The listing builds one solid part. Answer for the finished solid, in the listing's coordinates (mm). Give positions to 0.01 mm unless a question says otherwise; leave off trailing zeros. Loops run counter-clockwise (first coordinate to the right, second up) from the corner with the lowest first, then second, coordinate; pieces in that order, holes last.
Item 1: Consider line 1 along Z through (x, y) = (24.5, 1.4); line 2 along X through (y, z) = (2.2, 25); line 3 along Z through (x, y) = (26.5, 2). Determine where each line is inside the solid, lowest interval first.
Item 2: Section A-A, the plane z = -22 is taken. Give the vertices of the cut face in (x, y), and give its area (3 significant figures).
Item 3: Each of these flat-tipped pins is pushed along its axis until it touches: pin 1 Ø1 at (y, z) = (2.5, -5) entering from -X; pin 2 Ø2 at (y, z) = (2.5, 9.5) entering from +X; pin 3 Ø3 at (y, z) = (4, 6) entering from +X. Where does it stop, or does it pass through?
Item 4: Section C-C, the plane y = 3 is taken. Give the number of separate pieces and of enclosed holes in the cut face, and give its area (3 significant figures).
Item 5: The mould has two halves that part along Z. Classify faces 1 (the face through (-12.87, 2.58, -33.15)), 2 (the face through (-9, 5.08, -1)), 3 (the face through (-0.768, 2.576, -7.313)), 4 (the face through (29.18, 2.5, -31.83)): pulls with the +Z half, pulls with the -Z half, needs draft (parallel to the pull), parting line crosses it, or undercut.
Item 6: Section B-B, the plane x = 13 is taken. Give the vertices of the cut face in (y, z).
from build123d import *

# Parameters (mm, degrees)
SKETCH2_R           = 43.18
BOSS_EXTRUDE1_DEPTH = 5.08
CUT_EXTRUDE1_DEPTH  = 62.276677456
CUT_EXTRUDE2_DEPTH  = 62.276677456
SKETCH6_R           = 1.016
CUT_EXTRUDE3_DEPTH  = 62.276677456


with BuildPart() as part:
    # Sketch2 → Boss-Extrude1 (new body)
    with BuildSketch(Plane(origin=(0, 0, 0), x_dir=(1, 0, 0), z_dir=(0, 1, 0))):
        with Locations(Location((0, 0, 0), (0, 0, 270))):
            Circle(SKETCH2_R)
    extrude(amount=BOSS_EXTRUDE1_DEPTH)

    # Sketch3 → Cut-Extrude1 (cut, through all)
    with BuildSketch(Plane(origin=(0, 5.08, 0), x_dir=(1, 0, 0), z_dir=(0, 1, 0))):
        with BuildLine():
            Line((1.626393556, 2.3495), (-1.626393556, 2.3495))
            ThreePointArc((-1.626393556, 2.3495), (-1.326251609, -2.531079398), (2.8575, 0))
            ThreePointArc((2.8575, 0), (2.531079398, 1.326251609), (1.626393556, 2.3495))
        make_face()
    extrude(amount=-CUT_EXTRUDE1_DEPTH, mode=Mode.SUBTRACT)

    # Sketch5 → Cut-Extrude2 (cut, through all)
    with BuildSketch(Plane(origin=(0, 5.08, 0), x_dir=(1, 0, 0), z_dir=(0, 1, 0))):
        with BuildLine():
            Line((-9.058813318, 2.943386871), (-33.819569719, 10.98864432))
            ThreePointArc((-33.819569719, 10.98864432), (-35.492818655, -2.184816682), (-32.216498168, -15.053599097))
            Line((-32.216498168, -15.053599097), (-9.197962288, -2.474492827))
            ThreePointArc((-9.197962288, -2.474492827), (-9.521860059, 0.244552684), (-9.058813318, 2.943386871))
        make_face()
        with BuildLine():
            Line((-5.598654528, -7.705886871), (-20.901643572, -28.76864432))
            ThreePointArc((-20.901643572, -28.76864432), (-8.89, -34.430821948), (4.361378082, -35.291528463))
            Line((4.361378082, -35.291528463), (-0.488944133, -9.512442307))
            ThreePointArc((-0.488944133, -9.512442307), (-3.175, -8.980256121), (-5.598654528, -7.705886871))
        make_face()
        with BuildLine():
            Line((5.598654528, -7.705886871), (20.901643572, -28.76864432))
            ThreePointArc((20.901643572, -28.76864432), (29.9893062, -19.109032253), (34.905459287, -6.79135568))
            Line((34.905459287, -6.79135568), (8.894976784, -3.406613129))
            ThreePointArc((8.894976784, -3.406613129), (7.558920282, -5.795545631), (5.598654528, -7.705886871))
        make_face()
        with BuildLine():
            ThreePointArc((33.819569719, 10.98864432), (27.430090445, 22.629709193), (17.215410974, 31.115))
            Line((17.215410974, 31.115), (5.986837414, 7.408333333))
            ThreePointArc((5.986837414, 7.408333333), (7.847091067, 5.39896164), (9.058813318, 2.943386871))
            Line((9.058813318, 2.943386871), (33.819569719, 10.98864432))
        make_face()
        with BuildLine():
            ThreePointArc((0, 35.56), (-13.045768285, 33.080530979), (-24.272268948, 25.987892567))
            Line((-24.272268948, 25.987892567), (-5.195709188, 7.983121635))
            ThreePointArc((-5.195709188, 7.983121635), (-2.709833153, 9.131397992), (0, 9.525))
            Line((0, 9.525), (0, 35.56))
        make_face()
    extrude(amount=-CUT_EXTRUDE2_DEPTH, mode=Mode.SUBTRACT)

    # Sketch6 → Cut-Extrude3 (cut, through all)
    with BuildSketch(Plane(origin=(0, 5.08, 0), x_dir=(1, 0, 0), z_dir=(0, 1, 0))):
        with Locations(Location((5.738468444, 2.718911532, 0), (0, 0, 270))):
            Circle(SKETCH6_R)
        with Locations(Location((4.3591228, -4.617417938, 0), (0, 0, 270))):
            Circle(SKETCH6_R)
        with Locations(Location((-6.240654593, 1.173341487, 0), (0, 0, 270))):
            Circle(SKETCH6_R)
        with Locations(Location((-0.812554258, 6.297797677, 0), (0, 0, 270))):
            Circle(SKETCH6_R)
        with Locations(Location((-3.044382392, -5.572632757, 0), (0, 0, 270))):
            Circle(SKETCH6_R)
    extrude(amount=-CUT_EXTRUDE3_DEPTH, mode=Mode.SUBTRACT)


solid = part.part
Worked answers:
1. line 1: z = -35.56 to -25.77, -7.96 to 5.44, 25.77 to 35.56
1. line 2: x = -35.21 to -18.16, 2.43 to 18.16, 25.29 to 35.21
1. line 3: z = -34.09 to -23.71, -8.61 to 5.7, 23.71 to 34.09
2. outline: (-37.16, 0) - (-20.05, 0) - (-20.05, 5.08) - (-37.16, 5.08) - close; (0, 0) - (12.9, 0) - (12.9, 5.08) - (0, 5.08) - close; (27.94, 0) - (37.16, 0) - (37.16, 5.08) - (27.94, 5.08) - close
2. area: 199 mm2
3. pin 1: stops at x = -42.94
3. pin 2: stops at x = 42.34
3. pin 3: stops at x = 42.94
4. separate pieces: 1
4. enclosed holes: 11
4. area: 3,720 mm2
5. face 1: undercut
5. face 2: needs draft
5. face 3: undercut
5. face 4: parting line crosses it
6. outline: (0, -41.18) - (5.08, -41.18) - (5.08, -22.22) - (0, -22.22) - close; (0, -4.22) - (5.08, -4.22) - (5.08, 3.94) - (0, 3.94) - close; (0, 17.89) - (5.08, 17.89) - (5.08, 41.18) - (0, 41.18) - close
